Verification items for the finished model (mm, model axes). A direction names the side the tool comes from. Round coordinates to 2 decimals unless told otherwise and drop trailing zeros. Order: outer loops, then holes, each group sorted by start corner. A loop starts at its lowest first (then second) coordinate and runs counter-clockwise, first axis right, second up. Notation, with made-up numbers: (16, 63.5) -> (38, 63.5) arc R29 ccw to (38, 86.5) -> close; hole circle Ø7 at (50, -4.75). An arc over 180 degrees is marked (long way). Return JSON: item names as keys, results as strings. Group by question number.
Item 1: Scan lines: probe 1 along Y at (x, z) = (-18, 0.2); probe 2 along Y at (x, z) = (-18.75, 0.3); probe 3 along X at (y, z) = (18.5, 1.45). Record each from-to range of solid material in increasing order. Write a range as from..to.
Item 2: Sectioned sample at A-A on y = 17.75. Record the cut outline in (x, z).
Item 3: Sectioned sample at C-C on y = 2.5. Record the cut outline in (x, z).
Item 4: Access from +Z, -Z, +X, -X, +Y, -Y to the whole of each face (thin tool, end or side, straight path). Record for faces 1 (the flat face through (-18, 0, 1)), 2 (the cylindrical face through (-18.152, 28.587, 1.521)).
Item 5: Draft check along X on faces 3 (the flat face through (-22.117, 15, 1)), 4 (the flat face through (-19.705, 21, 2)), 5 (the flat face through (-14.117, 15, 1)), 6 (the flat face through (-16.53, 21, 2)). Enter one of: pulls with the +X half, pulls with the -X half, needs draft (parallel to the pull), parting line crosses it, or undercut.
Item 6: Sectioned sample at B-B on z = 0.5. Give the number of separate pieces and of enclosed holes in the cut face, plus the area to 3 significant figures.
Item 7: Depth check by flat-ended pin: pin 1 Ø4 at (x, y) = (-18.12, 2.5) entering from +Z. Enter the tip coordinate at first touch or a pass-through.
```python
from build123d import *

# Parameters (mm, degrees)
SKETCH1_W           = 8
SKETCH1_H           = 30
BOSS_EXTRUDE1_DEPTH = 3
SKETCH2_R           = 1.25
CUT_EXTRUDE1_DEPTH  = 3


with BuildPart() as part:
    # Sketch1 → Boss-Extrude1 (new body)
    with BuildSketch(Plane.XY):
        with Locations((-18.117004067, 15)):
            Rectangle(SKETCH1_W, SKETCH1_H)
    extrude(amount=BOSS_EXTRUDE1_DEPTH)

    # Sketch2 → Cut-Extrude1 (cut)
    with BuildSketch(Plane.XY.offset(3)):
        with Locations((-18.117004067, 2.5)):
            Circle(SKETCH2_R)
        with BuildLine():
            Line((-16.529504067, 27), (-16.529504067, 14.5))
            ThreePointArc((-16.529504067, 14.5), (-18.117004067, 12.9125), (-19.704504067, 14.5))
            Line((-19.704504067, 14.5), (-19.704504067, 27))
            ThreePointArc((-19.704504067, 27), (-18.117004067, 28.5875), (-16.529504067, 27))
        make_face()
    extrude(amount=-CUT_EXTRUDE1_DEPTH, mode=Mode.SUBTRACT)


solid = part.part
```
Recorded:
{
 "1": {"probe 1": "0..1.26, 3.74..12.92, 28.58..30", "probe 2": "0..1.42, 3.58..13.04, 28.46..30", "probe 3": "-22.12..-19.7, -16.53..-14.12"},
 "2": {"outline": "(-22.12, 0) -> (-19.7, 0) -> (-19.7, 3) -> (-22.12, 3) -> close; (-16.53, 0) -> (-14.12, 0) -> (-14.12, 3) -> (-16.53, 3) -> close"},
 "3": {"outline": "(-22.12, 0) -> (-19.37, 0) -> (-19.37, 3) -> (-22.12, 3) -> close; (-16.87, 0) -> (-14.12, 0) -> (-14.12, 3) -> (-16.87, 3) -> close"},
 "4": {"face 1": "+Z, -Z, +X, -X, -Y", "face 2": "+Z, -Z"},
 "5": {"face 3": "pulls with the -X half", "face 4": "undercut", "face 5": "pulls with the +X half", "face 6": "undercut"},
 "6": {"separate pieces": "1", "enclosed holes": "2", "area": "187 mm²"},
 "7": {"pin 1": "z = 3"}
}
